The listing builds one solid part. Answer for the finished solid, in the listing's coordinates (mm). A direction names the side the tool comes from. Round coordinates to 2 decimals unless told otherwise and drop trailing zeros. Loops run counter-clockwise (first coordinate to the right, second up) from the corner with the lowest first, then second, coordinate; pieces in that order, holes last. Notation, with made-up numbers: (-8, 58) -> (33, 58) arc R7 cw to (33, 69) -> close; hole circle Ø2 at (-24, 24). An arc over 180 degrees is marked (long way). Use a Markdown table: item, result. Add a question column.
Q1. Section A-A on x = 0 is taken. Give the vertices of the cut face in (y, z).
Q2. Which of the six approach directions +Z, -Z, +X, -X, +Y, -Y give full straight-line access (tool end or side, diameter ignored) to faces 1 (the cylindrical face through (-3.417, 76.52, -0.759)), 2 (the cylindrical face through (-3.417, 2.465, -0.759)), 3 (the flat face through (0, 147.5, 0))?
Q3. Given pin 1 Ø1 at (y, z) = (23.5, 2) entering from -X, flat-ended and moving along its own axis, determine where the tip first touches the part or whether it passes through.
Q4. Section C-C on y = 23 is taken. Give the vertices of the cut face in (x, z), then the cut area to 3 significant figures.
Q5. Consider line 1 (Y direction, x = 1.75, z = -3.5); line 2 (Z direction, x = -0.25, y = 120); line 3 (Z direction, x = 2.25, y = 71). Determine where each line is inside the solid, lowest interval first.
Q6. Section B-B on z = 0 is taken. Give the vertices of the cut face in (x, y), then the cut area to 4 significant figures.
from build123d import *

# Parameters (mm, degrees)
SKETCH1_R           = 3.5
BOSS_EXTRUDE1_DEPTH = 5
SKETCH2_R           = 4
BOSS_EXTRUDE2_DEPTH = 2.5
SKETCH3_R           = 3.5
BOSS_EXTRUDE3_DEPTH = 140


with BuildPart() as part:
    # Sketch1 → Boss-Extrude1 (new body)
    with BuildSketch(Plane(origin=(0, 0, 0), x_dir=(1, 0, 0), z_dir=(0, 1, 0))):
        with Locations(Location((0, 0, 0), (0, 0, 270))):  # turned: the seam where the file's is
            Circle(SKETCH1_R)
    extrude(amount=BOSS_EXTRUDE1_DEPTH)

    # Sketch2 → Boss-Extrude2 (add)
    with BuildSketch(Plane(origin=(0, 5, 0), x_dir=(1, 0, 0), z_dir=(0, 1, 0))):
        with Locations(Location((0, 0, 0), (0, 0, 270))):  # turned: the seam where the file's is
            Circle(SKETCH2_R)
    extrude(amount=BOSS_EXTRUDE2_DEPTH)

    # Sketch3 → Boss-Extrude3 (add)
    with BuildSketch(Plane(origin=(0, 7.5, 0), x_dir=(1, 0, 0), z_dir=(0, 1, 0))):
        with Locations(Location((0, 0, 0), (0, 0, 270))):  # turned: the seam where the file's is
            Circle(SKETCH3_R)
    extrude(amount=BOSS_EXTRUDE3_DEPTH)


solid = part.part
Checked values:
| question | item | result |
|---|---|---|
| 1 | outline | (0, -3.5) -> (5, -3.5) -> (5, -4) -> (7.5, -4) -> (7.5, -3.5) -> (147.5, -3.5) -> (147.5, 3.5) -> (7.5, 3.5) -> (7.5, 4) -> (5, 4) -> (5, 3.5) -> (0, 3.5) -> close |
| 2 | face 1 | +Y |
| 2 | face 2 | -Y |
| 2 | face 3 | +Z, -Z, +X, -X, +Y |
| 3 | pin 1 | stops at x = -3.16 |
| 4 | outline | circle Ø7 at (0, 0) |
| 4 | area | 38.5 mm2 |
| 5 | line 1 | y = 5 to 7.5 |
| 5 | line 2 | z = -3.49 to 3.49 |
| 5 | line 3 | z = -2.68 to 2.68 |
| 6 | outline | (-4, 5) -> (-3.5, 5) -> (-3.5, 0) -> (3.5, 0) -> (3.5, 5) -> (4, 5) -> (4, 7.5) -> (3.5, 7.5) -> (3.5, 147.5) -> (-3.5, 147.5) -> (-3.5, 7.5) -> (-4, 7.5) -> close |
| 6 | area | 1,035 mm2 |
